from build123d import *

# Parameters (mm, degrees)
SKETCH2_W           = 29
SKETCH2_H           = 19
BOSS_EXTRUDE1_DEPTH = 15
CUT_EXTRUDE1_DEPTH  = 13
SKETCH4_W           = 3
SKETCH4_H           = 5
CUT_EXTRUDE2_DEPTH  = 13
SKETCH5_W           = 33
SKETCH5_H           = 23
BOSS_EXTRUDE2_DEPTH = 2
FILLET1_R           = 5
FILLET2_R           = 5
FILLET3_R           = 5
FILLET4_R           = 5


with BuildPart() as part:
    # Sketch2 → Boss-Extrude1 (new body)
    with BuildSketch(Plane(origin=(0, 0, 0), x_dir=(1, 0, 0), z_dir=(0, 1, 0))):
        with Locations((12.5, 7.5)):
            Rectangle(SKETCH2_W, SKETCH2_H)
    extrude(amount=BOSS_EXTRUDE1_DEPTH)

    # Sketch3 → Cut-Extrude1 (cut)
    with BuildSketch(Plane.XZ):
        Polygon((0, 0), (0, -10), (5, -15), (20, -15), (25, -10), (25, 0), align=None)
    extrude(amount=-CUT_EXTRUDE1_DEPTH, mode=Mode.SUBTRACT)

    # Sketch4 → Cut-Extrude2 (cut)
    with BuildSketch(Plane.XZ.offset(-13)):
        with Locations((4.5, -5.5)):
            Rectangle(SKETCH4_W, SKETCH4_H)
        with Locations((12.5, -9.5)):
            Rectangle(SKETCH4_W, SKETCH4_H)
        with Locations((20.5, -5.5)):
            Rectangle(SKETCH4_W, SKETCH4_H)
    extrude(amount=-CUT_EXTRUDE2_DEPTH, mode=Mode.SUBTRACT)

    # Sketch5 → Boss-Extrude2 (add)
    with BuildSketch(Plane.XZ):
        with Locations((12.5, -7.5)):
            Rectangle(SKETCH5_W, SKETCH5_H)
        Polygon((0, 0), (0, -10), (5, -15), (20, -15), (25, -10), (25, 0), align=None, mode=Mode.SUBTRACT)
    extrude(amount=BOSS_EXTRUDE2_DEPTH)

    # Fillet1
    fillet1_edges = [part.edges().sort_by_distance(p)[0] for p in [
        (29, -1, -19),
    ]]
    fillet(fillet1_edges, radius=FILLET1_R)

    # Fillet2
    fillet2_edges = [part.edges().sort_by_distance(p)[0] for p in [
        (29, -1, 4),
    ]]
    fillet(fillet2_edges, radius=FILLET2_R)

    # Fillet3
    fillet3_edges = [part.edges().sort_by_distance(p)[0] for p in [
        (-4, -1, 4),
    ]]
    fillet(fillet3_edges, radius=FILLET3_R)

    # Fillet4
    fillet4_edges = [part.edges().sort_by_distance(p)[0] for p in [
        (-4, -1, -19),
    ]]
    fillet(fillet4_edges, radius=FILLET4_R)


solid = part.part
Geometry: final body of the model. Coordinates: model frame, mm. A direction names the side the tool comes from. Give positions to 0.01 mm unless a question says otherwise; leave off trailing zeros. Loops run counter-clockwise (first coordinate to the right, second up) from the corner with the lowest first, then second, coordinate; pieces in that order, holes last. Notation, with made-up numbers: M 1,-5.5 L 59,-5.5 A21 ccw 59,20.5 Z; hole C 85,-39 d1. An arc over 180 degrees is marked long. Put each result on its own line as item: value.
1) Cut plane B-B, the plane z = -5.75. Return the cut outline in (x, y), plus the area to 3 significant figures.
Computed values:
outline: M -4,-2 L 0,-2 L 0,13 L 3,13 L 3,15 L -2,15 L -2,0 L -4,0 Z; M 6,13 L 19,13 L 19,15 L 6,15 Z; M 22,13 L 25,13 L 25,-2 L 29,-2 L 29,0 L 27,0 L 27,15 L 22,15 Z
area: 114 mm^2
2) Cut plane C-C, the plane y = 8.5. Return the cut outline in (x, z).
Computed values:
outline: M -2,-17 L 27,-17 L 27,2 L -2,2 Z; hole M 0,-10 L 5,-15 L 20,-15 L 25,-10 L 25,0 L 0,0 Z
3) Reachability of faces 4 (the flat face through (12, -1, -19)), 5 (the flat face through (-2, 7, -7)), 6 (the flat face through (0, 6, -5)), 7 (the flat face through (12, 7, -17)), 8 (the flat face through (12, 14, -7)) from +Z, -Z, +X, -X, +Y, -Y: full face, straight path, thin tool, end or side. Return the list, or none.
Computed values:
face 4: -Z, +X, -X, +Y, -Y
face 5: +Z, -Z, -X, +Y
face 6: -Y
face 7: -Z, +X, -X, +Y
face 8: +Y, -Y
4) First-contact query: P1, Ø2, axis at x = 4, y = 14, coming from the +Z side; P2, Ø3, axis at x = 24, y = 6.5, coming from the -Z side; P3, Ø7.5, axis at y = 5.5, z = -9, coming from the -X side. Flat tips, straight axial feed; report the tip coordinate or a pass-through.
Computed values:
P1: stops at z = 2
P2: stops at z = -17
P3: stops at x = -2
5) Mould query, pull axis Z, two halves, no side actions, for faces 1 (the flat face through (12, 7, 2)), 2 (the flat face through (29, -1, -8)), 3 (the flat face through (3, 14, -6)). Classes: released by +Z, released by -Z, zero draft, split by the parting line, or undercut.
Computed values:
face 1: released by +Z
face 2: zero draft
face 3: undercut
6) Cut plane D-D, the plane x = 23. Return the cut outline in (y, z).
Computed values:
outline: M -2,-19 L 0,-19 L 0,-17 L 15,-17 L 15,2 L 0,2 L 0,4 L -2,4 L -2,0 L 13,0 L 13,-12 L -2,-12 Z
7) Material intervals for L1, parallel to X at y = -1.5, z = -8.25; L2, parallel to Z at x = 9, y = 3; L3, parallel to X at y = 12.75, z = -7, sorted ascending. Write a range as from..to.
Computed values:
L1: x = -4..0, 25..29
L2: z = -17..-15, 0..2
L3: x = -2..0, 25..27
8) Cut plane A-A, the plane x = 19.5. Return the cut outline in (y, z), plus the area to 3 significant figures.
Computed values:
outline: M -2,-19 L 0,-19 L 0,-17 L 15,-17 L 15,-8 L 13,-8 L 13,-15 L -2,-15 Z; M -2,0 L 13,0 L 13,-3 L 15,-3 L 15,2 L 0,2 L 0,4 L -2,4 Z
area: 96.0 mm^2
